```python
from build123d import *

# Parameters (mm, degrees)
SKETCH1_R           = 63.5
SKETCH1_R_2         = 76.2
SKETCH1_R_3         = 127
SKETCH1_R_4         = 101.6
SKETCH1_R_5         = 254
SKETCH1_W           = 1270
SKETCH1_H           = 1270
BOSS_EXTRUDE1_DEPTH = 50
SCALE1_SCALE        = 0.04


with BuildPart() as part:
    # Sketch1 → Boss-Extrude1 (new body)
    with BuildSketch(Plane.XY):
        Polygon((50.8, 3435.35), (50.8, 3956.05), (0, 3956.05), (0, 4476.75), (50.8, 4476.75), (50.8, 4997.45), (0, 4997.45), (0, 5518.15), (50.8, 5518.15), (50.8, 6299.2), (539.75, 6299.2), (539.75, 6350), (1060.45, 6350), (1060.45, 6299.2), (1581.15, 6299.2), (1581.15, 6350), (2101.85, 6350), (2101.85, 6299.2), (2622.55, 6299.2), (2622.55, 6350), (3143.25, 6350), (3143.25, 6299.2), (3663.95, 6299.2), (3663.95, 6350), (4184.65, 6350), (4184.65, 6299.2), (4705.35, 6299.2), (4705.35, 6350), (5226.05, 6350), (5226.05, 6299.2), (5746.75, 6299.2), (5746.75, 6350), (6267.45, 6350), (6267.45, 6299.2), (6788.15, 6299.2), (6788.15, 6350), (7308.85, 6350), (7308.85, 6299.2), (7829.55, 6299.2), (7829.55, 6350), (8350.25, 6350), (8350.25, 6299.2), (8839.2, 6299.2), (8839.2, 6038.85), (8839.2, 5518.15), (8890, 5518.15), (8890, 4997.45), (8839.2, 4997.45), (8839.2, 4476.75), (8890, 4476.75), (8890, 3956.05), (8839.2, 3956.05), (8839.2, 3435.35), (8890, 3435.35), (8890, 2914.65), (8839.2, 2914.65), (8839.2, 2393.95), (8890, 2393.95), (8890, 1873.25), (8839.2, 1873.25), (8839.2, 1352.55), (8890, 1352.55), (8890, 831.85), (8839.2, 831.85), (8839.2, 50.8), (8350.25, 50.8), (8350.25, 0), (7829.55, 0), (7829.55, 50.8), (7308.85, 50.8), (7308.85, 0), (6788.15, 0), (6788.15, 50.8), (6267.45, 50.8), (6267.45, 0), (5746.75, 0), (5746.75, 50.8), (5226.05, 50.8), (5226.05, 0), (4705.35, 0), (4705.35, 50.8), (4184.65, 50.8), (4184.65, 0), (3663.95, 0), (3663.95, 50.8), (3143.25, 50.8), (3143.25, 0), (2622.55, 0), (2622.55, 50.8), (2101.85, 50.8), (2101.85, 0), (1581.15, 0), (1581.15, 50.8), (1060.45, 50.8), (1060.45, 0), (539.75, 0), (539.75, 50.8), (50.8, 50.8), (50.8, 311.15), (50.8, 831.85), (0, 831.85), (0, 1352.55), (50.8, 1352.55), (50.8, 1873.25), (0, 1873.25), (0, 2393.95), (50.8, 2393.95), (50.8, 2914.65), (0, 2914.65), (0, 3435.35), align=None)
        with Locations((2263.093189832, 4514.095537704)):
            Circle(SKETCH1_R, mode=Mode.SUBTRACT)
        with Locations((7182.429020432, 5834.895537704)):
            Circle(SKETCH1_R_2, mode=Mode.SUBTRACT)
        with Locations((6147.900253832, 5834.895537704)):
            Circle(SKETCH1_R_2, mode=Mode.SUBTRACT)
        with Locations((8071.429020432, 5834.895537704)):
            Circle(SKETCH1_R_2, mode=Mode.SUBTRACT)
        with Locations((3988.900253832, 5834.895537704)):
            Circle(SKETCH1_R_2, mode=Mode.SUBTRACT)
        with Locations((993.093189832, 5784.095537704)):
            Circle(SKETCH1_R_3, mode=Mode.SUBTRACT)
        with Locations((993.093189832, 5149.095537704)):
            Circle(SKETCH1_R_4, mode=Mode.SUBTRACT)
        with Locations((993.093189832, 4514.095537704)):
            Circle(SKETCH1_R, mode=Mode.SUBTRACT)
        with Locations((1501.093189832, 5784.095537704)):
            Circle(SKETCH1_R_3, mode=Mode.SUBTRACT)
        with Locations((1501.093189832, 5149.095537704)):
            Circle(SKETCH1_R_4, mode=Mode.SUBTRACT)
        with Locations((1501.093189832, 4514.095537704)):
            Circle(SKETCH1_R, mode=Mode.SUBTRACT)
        with Locations((2263.093189832, 5784.095537704)):
            Circle(SKETCH1_R_5, mode=Mode.SUBTRACT)
        with Locations((2263.093189832, 5149.095537704)):
            Circle(SKETCH1_R_4, mode=Mode.SUBTRACT)
        with Locations((2739.3392, 3152.6226)):
            Rectangle(SKETCH1_W, SKETCH1_H, mode=Mode.SUBTRACT)
        with Locations((2739.3392, 1755.6226)):
            Rectangle(SKETCH1_W, SKETCH1_H, mode=Mode.SUBTRACT)
        with Locations((1342.3392, 1755.6226)):
            Rectangle(SKETCH1_W, SKETCH1_H, mode=Mode.SUBTRACT)
        with Locations((1342.3392, 3152.6226)):
            Rectangle(SKETCH1_W, SKETCH1_H, mode=Mode.SUBTRACT)
    extrude(amount=BOSS_EXTRUDE1_DEPTH)


with BuildPart() as part_1:
    # Scale1: scaled about (4784.759817545, 3245.327855947, 25)
    add(part.part.scale(SCALE1_SCALE).moved(Location((4593.369424843, 3115.514741709, 24))))


solid = part_1.part
```
Source: CAD feature listing. Evaluate the final solid. Frame: model axes, mm. Give positions to 0.01 mm unless a question says otherwise; leave off trailing zeros. Loops run counter-clockwise (first coordinate to the right, second up) from the corner with the lowest first, then second, coordinate; pieces in that order, holes last. Notation, with made-up numbers: (-12, -15) -> (45, -15) arc R29 ccw to (45, 20) -> close; hole circle Ø3 at (0, 7.25). An arc over 180 degrees is marked (long way). Put each result on its own line as item: value. Start each with the question number.
1) Cut plane A-A (x = 4902). Return loops of the section in (y, z).
2) Cut plane B-B (z = 25.5). State how many separate pieces and enclosed holes the cut face has, then the cut area to 3 significant figures.
3) Material intervals for probe 1 along Y at (x, z) = (4664.5, 25.05); probe 2 along X at (y, z) = (3321, 25.2); probe 3 along X at (y, z) = (3263.5, 24.6), sorted ascending.
4) Contact query for flat-ended pins moving along their axis: P1, Ø1, axis at x = 4858, z = 25, coming from the -Y side; P2, Ø1, axis at y = 3178, z = 24.5, coming from the -X side; P3, Ø4.5, axis at x = 4683.89, y = 3296.08, coming from the -Z side; P4, Ø10.5, axis at x = 4633.09, y = 3321.48, coming from the -Z side. Output: stop coordinate, or through.
5) Draft query along X for faces 1 (the face through (4774, 3244, 24)), 2 (the face through (4693.28, 3342.99, 24.99)), 3 (the face through (4648.338, 3347.102, 24.986)). Return one class per face: released by +X, released by -X, zero draft, split by the parting line, or undercut.
Results are:
1. outline: (3117.55, 24) -> (3367.48, 24) -> (3367.48, 26) -> (3117.55, 26) -> close
2. separate pieces: 1
2. enclosed holes: 17
2. area: 77,800 mm2
3. probe 1: y = 3115.51 to 3160.34, 3211.14 to 3216.22, 3267.02 to 3369.51
3. probe 2: x = 4593.37 to 4629.06, 4637.13 to 4649.38, 4657.45 to 4679.86, 4687.93 to 4948.97
3. probe 3: x = 4595.4 to 4621.66, 4672.46 to 4677.54, 4728.34 to 4946.94
4. P1: stops at y = 3117.55
4. P2: stops at x = 4595.4
4. P3: passes through
4. P4: stops at z = 24
5. face 1: zero draft
5. face 2: undercut
5. face 3: undercut
